from build123d import *

# Parameters (mm, degrees)
BOSS_EXTRUDE1_DEPTH = 457.2
SKETCH2_W           = 136.525
SKETCH2_H           = 4.7625
CUT_EXTRUDE1_DEPTH  = 479.481428682
SKETCH3_W           = 132.265960651
SKETCH3_H           = 13.462
CUT_EXTRUDE2_DEPTH  = 479.481428682
SKETCH9_OUTSIDE_W   = 234.019
SKETCH9_OUTSIDE_H   = 554.694
SKETCH9_OUTSIDE_W_2 = 94.360380141
SKETCH9_OUTSIDE_H_2 = 481.67440371
CUT_EXTRUDE3_DEPTH  = 478.468171223


with BuildPart() as part:
    # Sketch1 → Boss-Extrude1 (new body)
    with BuildSketch(Plane(origin=(0, 0, 0), x_dir=(1, 0, 0), z_dir=(0, 1, 0))):
        with BuildLine():
            Line((0, 0), (136.525, 0))
            Line((136.525, 0), (136.525, 9.525))
            Line((136.525, 9.525), (132.5372, 9.525))
            Line((132.5372, 9.525), (132.5372, 34.925))
            ThreePointArc((132.5372, 34.925), (131.7752, 35.687), (131.0132, 34.925))
            Line((131.0132, 34.925), (131.0132, 9.525))
            Line((131.0132, 9.525), (126.1872, 9.525))
            Line((126.1872, 9.525), (126.1872, 34.925))
            ThreePointArc((126.1872, 34.925), (125.4252, 35.687), (124.6632, 34.925))
            Line((124.6632, 34.925), (124.6632, 9.525))
            Line((124.6632, 9.525), (119.8372, 9.525))
            Line((119.8372, 9.525), (119.8372, 34.925))
            ThreePointArc((119.8372, 34.925), (119.0752, 35.687), (118.3132, 34.925))
            Line((118.3132, 34.925), (118.3132, 9.525))
            Line((118.3132, 9.525), (113.4872, 9.525))
            Line((113.4872, 9.525), (113.4872, 34.925))
            ThreePointArc((113.4872, 34.925), (112.7252, 35.687), (111.9632, 34.925))
            Line((111.9632, 34.925), (111.9632, 9.525))
            Line((111.9632, 9.525), (107.1372, 9.525))
            Line((107.1372, 9.525), (107.1372, 34.925))
            ThreePointArc((107.1372, 34.925), (106.3752, 35.687), (105.6132, 34.925))
            Line((105.6132, 34.925), (105.6132, 9.525))
            Line((105.6132, 9.525), (100.7872, 9.525))
            Line((100.7872, 9.525), (100.7872, 34.925))
            ThreePointArc((100.7872, 34.925), (100.0252, 35.687), (99.2632, 34.925))
            Line((99.2632, 34.925), (99.2632, 9.525))
            Line((99.2632, 9.525), (94.4372, 9.525))
            Line((94.4372, 9.525), (94.4372, 34.925))
            ThreePointArc((94.4372, 34.925), (93.6752, 35.687), (92.9132, 34.925))
            Line((92.9132, 34.925), (92.9132, 9.525))
            Line((92.9132, 9.525), (88.0872, 9.525))
            Line((88.0872, 9.525), (88.0872, 34.925))
            ThreePointArc((88.0872, 34.925), (87.3252, 35.687), (86.5632, 34.925))
            Line((86.5632, 34.925), (86.5632, 9.525))
            Line((86.5632, 9.525), (81.7372, 9.525))
            Line((81.7372, 9.525), (81.7372, 34.925))
            ThreePointArc((81.7372, 34.925), (80.9752, 35.687), (80.2132, 34.925))
            Line((80.2132, 34.925), (80.2132, 9.525))
            Line((80.2132, 9.525), (75.3872, 9.525))
            Line((75.3872, 9.525), (75.3872, 34.925))
            ThreePointArc((75.3872, 34.925), (74.6252, 35.687), (73.8632, 34.925))
            Line((73.8632, 34.925), (73.8632, 9.525))
            Line((73.8632, 9.525), (69.0372, 9.525))
            Line((69.0372, 9.525), (69.0372, 34.925))
            ThreePointArc((69.0372, 34.925), (68.2752, 35.687), (67.5132, 34.925))
            Line((67.5132, 34.925), (67.5132, 9.525))
            Line((67.5132, 9.525), (62.6872, 9.525))
            Line((62.6872, 9.525), (62.6872, 34.925))
            ThreePointArc((62.6872, 34.925), (61.9252, 35.687), (61.1632, 34.925))
            Line((61.1632, 34.925), (61.1632, 9.525))
            Line((61.1632, 9.525), (56.3372, 9.525))
            Line((56.3372, 9.525), (56.3372, 34.925))
            ThreePointArc((56.3372, 34.925), (55.5752, 35.687), (54.8132, 34.925))
            Line((54.8132, 34.925), (54.8132, 9.525))
            Line((54.8132, 9.525), (49.9872, 9.525))
            Line((49.9872, 9.525), (49.9872, 34.925))
            ThreePointArc((49.9872, 34.925), (49.2252, 35.687), (48.4632, 34.925))
            Line((48.4632, 34.925), (48.4632, 9.525))
            Line((48.4632, 9.525), (43.6372, 9.525))
            Line((43.6372, 9.525), (43.6372, 34.925))
            ThreePointArc((43.6372, 34.925), (42.8752, 35.687), (42.1132, 34.925))
            Line((42.1132, 34.925), (42.1132, 9.525))
            Line((42.1132, 9.525), (37.2872, 9.525))
            Line((37.2872, 9.525), (37.2872, 34.925))
            ThreePointArc((37.2872, 34.925), (36.5252, 35.687), (35.7632, 34.925))
            Line((35.7632, 34.925), (35.7632, 9.525))
            Line((35.7632, 9.525), (30.9372, 9.525))
            Line((30.9372, 9.525), (30.9372, 34.925))
            ThreePointArc((30.9372, 34.925), (30.1752, 35.687), (29.4132, 34.925))
            Line((29.4132, 34.925), (29.4132, 9.525))
            Line((29.4132, 9.525), (24.5872, 9.525))
            Line((24.5872, 9.525), (24.5872, 34.925))
            ThreePointArc((24.5872, 34.925), (23.8252, 35.687), (23.0632, 34.925))
            Line((23.0632, 34.925), (23.0632, 9.525))
            Line((23.0632, 9.525), (18.2372, 9.525))
            Line((18.2372, 9.525), (18.2372, 34.925))
            ThreePointArc((18.2372, 34.925), (17.4752, 35.687), (16.7132, 34.925))
            Line((16.7132, 34.925), (16.7132, 9.525))
            Line((16.7132, 9.525), (11.8872, 9.525))
            Line((11.8872, 9.525), (11.8872, 34.925))
            ThreePointArc((11.8872, 34.925), (11.1252, 35.687), (10.3632, 34.925))
            Line((10.3632, 34.925), (10.3632, 9.525))
            Line((10.3632, 9.525), (5.5372, 9.525))
            Line((5.5372, 9.525), (5.5372, 34.925))
            ThreePointArc((5.5372, 34.925), (4.7752, 35.687), (4.0132, 34.925))
            Line((4.0132, 34.925), (4.0132, 9.525))
            Line((4.0132, 9.525), (0, 9.525))
            Line((0, 9.525), (0, 0))
        make_face()
    extrude(amount=BOSS_EXTRUDE1_DEPTH)

    # Sketch2 → Cut-Extrude1 (cut, through all)
    with BuildSketch(Plane(origin=(0, 457.2, 0), x_dir=(1, 0, 0), z_dir=(0, 1, 0))):
        with Locations((68.2625, 2.38125)):
            Rectangle(SKETCH2_W, SKETCH2_H)
    extrude(amount=-CUT_EXTRUDE1_DEPTH, mode=Mode.SUBTRACT)

    # Sketch3 → Cut-Extrude2 (cut, through all)
    with BuildSketch(Plane.XZ):
        with Locations((69.2831702, -28.956)):
            Rectangle(SKETCH3_W, SKETCH3_H)
    extrude(amount=-CUT_EXTRUDE2_DEPTH, mode=Mode.SUBTRACT)

    # Sketch9 outside → Cut-Extrude3 (cut, through all)
    with BuildSketch(Plane.XY.offset(-4.7625)):
        with Locations((68.2625, 228.6)):
            Rectangle(SKETCH9_OUTSIDE_W, SKETCH9_OUTSIDE_H)
        with Locations((68.07230993, 238.432707494)):
            Rectangle(SKETCH9_OUTSIDE_W_2, SKETCH9_OUTSIDE_H_2, mode=Mode.SUBTRACT)
    extrude(amount=-CUT_EXTRUDE3_DEPTH, mode=Mode.SUBTRACT)


solid = part.part
Read the model definition and answer for the solid it produces. Units are mm, in the model's axes. A direction names the side the tool comes from. Round coordinates to 2 decimals unless told otherwise and drop trailing zeros. Use one line per item in the form item = value. Start each with the question number.
(1) Flat-ended cylindrical pins translate along their axes: pin 1 Ø2.5 at (x, y) = (78.5, 141) entering from -Z (3 decimals); pin 2 Ø4 at (y, z) = (237.5, -16) entering from +X; pin 3 Ø4 at (y, z) = (215.5, -17.5) entering from -X. Find the tip coordinate at first contact, or state that the pin passes through.
(2) For faces 4 (the face through (107.137, 225, -16)), 5 (the face through (67, 232, -4.762)), determine the directions among +Z, -Z, +X, -X, +Y, -Y from which every point of the face is accessible in a straight line to the end or side of a thin tool.
(3) Determine the mould class of faces 1 (the face through (23.063, 225, -16)), 2 (the face through (71, 0, -8)), 3 (the face through (105.613, 225, -16)) for opening direction X: +X half, -X half, draft (parallel to the pull), parting line (faces both ways), or undercut.
(4) Find the intervals of material crossed by line 1 along Z through (x, y) = (35.5, 160) (1 decimal), in increasing order. Write a range as from..to.
(5) The part is cut by section A-A (z = -17.5). Count the separate pieces of the cut face and the enclosed holes in it, then the cut area to 3 significant figures.
Checked values:
q1.pin_1 = -9.525
q1.pin_2 = 113.49
q1.pin_3 = 23.06
q2.face_4 = -Z, +Y, -Y
q2.face_5 = +Z, +X, -X, +Y, -Y
q3.face_1 = -X half
q3.face_2 = draft
q3.face_3 = undercut
q4.line_1 = -9.5..-4.8
q5.separate_pieces = 15
q5.enclosed_holes = 0
q5.area = 10,500 mm^2
